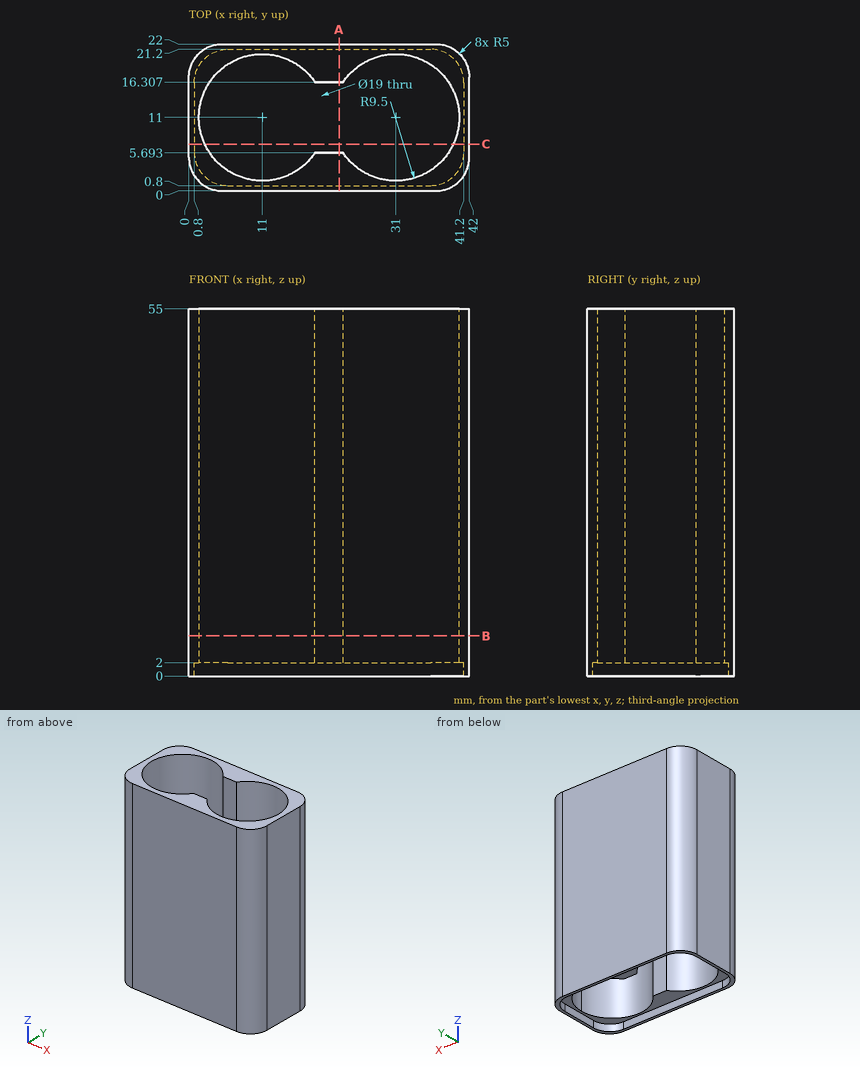
Study the drawing (mm; zero at the part's minimum x, y, z) and answer. Give positions to 0.01 mm unless a question says otherwise; leave off trailing zeros. Loops run counter-clockwise (first coordinate to the right, second up) from the corner with the lowest first, then second, coordinate; pieces in that order, holes last. Notation, with made-up numbers: M 24.5,78 L 50.5,78 A22 ccw 50.5,107 Z; hole C 62.5,69 d1. An arc over 180 degrees is marked long. One line per item, written item: value.
1. Find the intervals of material crossed by probe 1 along Y at (x, z) = (11, 30); probe 2 along X at (y, z) = (2.5, 10) (1 decimal); probe 3 along Y at (x, z) = (21, 45.5), in increasing order.
Found:
probe 1: 0 to 1.5, 20.5 to 22
probe 2: 0.7 to 6.8, 15.2 to 26.8, 35.2 to 41.3
probe 3: 0 to 5.69, 16.31 to 22
2. Section B-B on z = 6 is taken. Determine the outline of the cut face in (x, y), plus the area to 3 significant figures.
Found:
outline: M 0,5 A5 ccw 5,0 L 37,0 A5 ccw 42,5 L 42,17 A5 ccw 37,22 L 5,22 A5 ccw 0,17 Z; hole M 18.88,5.69 L 23.12,5.69 A9.5 ccw long 23.12,16.31 L 18.88,16.31 A9.5 ccw long Z
area: 314 mm^2
3. Section C-C on y = 7 is taken. Determine the outline of the cut face in (x, z), plus the area to 3 significant figures.
Found:
outline: M 0,0 L 0.8,0 L 0.8,2 L 2.38,2 L 2.38,55 L 0,55 Z; M 39.62,2 L 41.2,2 L 41.2,0 L 42,0 L 42,55 L 39.62,55 Z
area: 256 mm^2
4. Section A-A on x = 22.5 is taken. Determine the outline of the cut face in (y, z), plus the area to 3 significant figures.
Found:
outline: M 0,0 L 0.8,0 L 0.8,2 L 5.69,2 L 5.69,55 L 0,55 Z; M 16.31,2 L 21.2,2 L 21.2,0 L 22,0 L 22,55 L 16.31,55 Z
area: 607 mm^2
5. Each of these flat-tipped pins is pushed along its axis until it touches: P1, Ø8, axis at x = 33.5, y = 7.5, coming from the -Z side; P2, Ø1.3, axis at x = 21, z = 19, coming from the -Y side; P3, Ø5, axis at x = 15.5, y = 18.5, coming from the -Z side. Where does it stop, or does it pass through?
Found:
P1: through
P2: y = 0
P3: z = 2
